Could you check a few things on this model? Use its own coordinates, in mm. Face numbers are marked on the shaded views. A direction names the side the tool comes from. Coordinates: 2 decimals unless noted, no trailing zeros. Loops run counter-clockwise (first coordinate to the right, second up) from the corner with the lowest first, then second, coordinate; pieces in that order, holes last. Notation, with made-up numbers: M 78,33 L 128,33 A16 cw 128,45 Z; hole C -5.5,-36.5 d11. An arc over 180 degrees is marked long. Use one line per item in the form item = value. Start each with the question number.
```python
from build123d import *

# Parameters (mm, degrees)
F0_R     = 10.5
F1_DEPTH = 6.35


with BuildPart() as f1:
    # F0 (on Top) → F1 (new body)
    with BuildSketch(Plane.XY):
        with BuildLine():
            ThreePointArc((6.44846, 29.992483), (-15.414201, 40.590403), (-10.190932, 16.862585))
            ThreePointArc((-10.190932, 16.862585), (-3.961799, 16.850813), (1.609508, 19.63699))
            ThreePointArc((1.609508, 19.63699), (5.17904, 24.277334), (6.44846, 29.992483))
        make_face()
        with Locations((-7.05154, 29.992483)):
            Circle(F0_R, mode=Mode.SUBTRACT)
        with BuildLine():
            Line((-14.895684, -5.7813), (-6.689736, -14.510419))
            ThreePointArc((-6.689736, -14.510419), (3.65694, -15.554151), (12.454594, -10.00939))
            Line((12.454594, -10.00939), (16.201378, -11.21237))
            ThreePointArc((16.201378, -11.21237), (16.574131, -4.994388), (19.698893, 0.394313))
            Line((19.698893, 0.394313), (15.911259, 1.461728))
            ThreePointArc((15.911259, 1.461728), (11.64182, 10.944078), (2.441089, 15.79069))
            Line((2.441089, 15.79069), (1.609508, 19.63699))
            ThreePointArc((1.609508, 19.63699), (-3.961799, 16.850813), (-10.190932, 16.862585))
            Line((-10.190932, 16.862585), (-9.221523, 13.048691))
            ThreePointArc((-9.221523, 13.048691), (-15.29876, 4.610072), (-14.895684, -5.7813))
        make_face()
        Circle(F0_R, mode=Mode.SUBTRACT)
        with BuildLine():
            Line((-9.507961, -17.256899), (-6.689736, -14.510419))
            Line((-6.689736, -14.510419), (-14.895684, -5.7813))
            Line((-14.895684, -5.7813), (-17.810886, -8.42462))
            ThreePointArc((-17.810886, -8.42462), (-12.612333, -11.856425), (-9.507961, -17.256899))
        make_face()
        with BuildLine():
            ThreePointArc((19.698893, 0.394313), (16.574131, -4.994388), (16.201378, -11.21237))
            ThreePointArc((16.201378, -11.21237), (30.665848, -22.338996), (43.000022, -8.889429))
            ThreePointArc((43.000022, -8.889429), (34.496759, 3.651808), (19.698893, 0.394313))
        make_face()
        with Locations((29.500022, -8.889429)):
            Circle(F0_R, mode=Mode.SUBTRACT)
        with BuildLine():
            ThreePointArc((-8.948482, -21.103054), (-9.089084, -19.159737), (-9.507961, -17.256899))
            ThreePointArc((-9.507961, -17.256899), (-12.612333, -11.856425), (-17.810886, -8.42462))
            ThreePointArc((-17.810886, -8.42462), (-33.513236, -28.837472), (-8.948482, -21.103054))
        make_face()
        with Locations((-22.448482, -21.103054)):
            Circle(F0_R, mode=Mode.SUBTRACT)
    extrude(amount=F1_DEPTH)


solid = f1.part
```
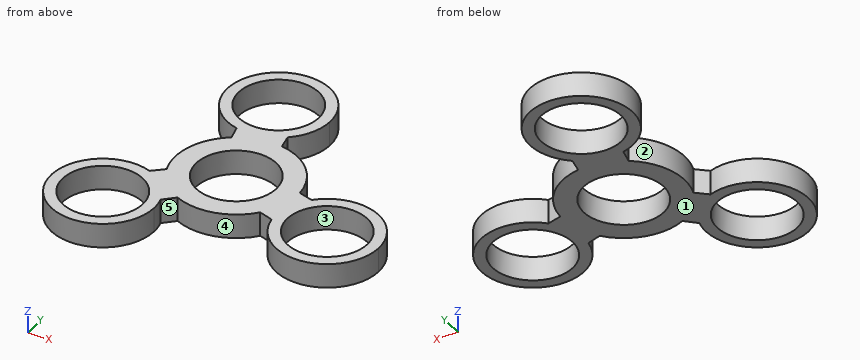
Item 1: I want a section at C-C (z = 4.5). Write out the boundary of the cut face in (x, y), plus the area to 3 significant figures.
Item 2: Thinking about a two-plate mould opening in X: for the marked faces 1, 2 and 3, which applies, pulls with the +X half, pulls with the -X half, needs draft (parallel to the pull), parting line crosses it, or undercut?
Item 3: I'm going to push flat-ended pins straight in: P1, Ø17, axis at x = -22.45, y = -21.1, coming from the +Z side; P2, Ø3, axis at y = -10, z = 4, coming from the -X side; P3, Ø1, axis at y = 11, z = 0.5, coming from the -X side. Where does each tip first touch, or does it pass through?
Item 4: I want a section at D-D (x = 0). Write out the boundary of the cut face in (y, z).
Item 5: I want a section at B-B (y = 28.5). Write out the boundary of the cut face in (x, z), plus the area to 3 significant figures.
Item 6: For the marked faces 4 and 5, which set-ups out of +Z, -Z, +X, -X, +Y, -Y let a thin tool reach every point of the face, with its end or its side?
Item 7: I want a section at A-A (x = 29.5). Write out the boundary of the cut face in (y, z), plus the area to 3 significant figures.
Item 8: Please list where these lines run through material, in increasing order: line 1 along Y through (x, z) = (-6, 6); line 2 along Y through (x, z) = (-1, 3.75); line 3 along X through (y, z) = (-20.5, 4.5) (3 decimals).
Worked answers:
q1.outline = M -17.81,-8.42 A13.5 ccw long -9.51,-17.26 L -6.69,-14.51 A15.98 ccw 12.45,-10.01 L 16.2,-11.21 A13.5 ccw long 19.7,0.39 L 15.91,1.46 A15.98 ccw 2.44,15.79 L 1.61,19.64 A13.5 ccw 6.45,29.99 A13.5 ccw long -10.19,16.86 L -9.22,13.05 A15.98 ccw -14.9,-5.78 Z; hole C -22.45,-21.1 d21; hole C -7.05,29.99 d21; hole C 0,0 d21; hole C 29.5,-8.89 d21
q1.area = 1,210 mm²
q2.face_1 = needs draft
q2.face_2 = pulls with the -X half
q2.face_3 = undercut
q3.P1 = through
q3.P2 = -31.94
q3.P3 = -12.04
q4.outline = M -15.98,0 L -10.5,0 L -10.5,6.35 L -15.98,6.35 Z; M 10.5,0 L 22.21,0 L 22.21,6.35 L 10.5,6.35 Z; M 37.77,0 L 41.5,0 L 41.5,6.35 L 37.77,6.35 Z
q5.outline = M -20.47,0 L -17.44,0 L -17.44,6.35 L -20.47,6.35 Z; M 3.34,0 L 6.37,0 L 6.37,6.35 L 3.34,6.35 Z
q5.area = 38.4 mm²
q6.face_4 = +Z, -Z, -Y
q6.face_5 = +Z, -Z
q7.outline = M -22.39,0 L -19.39,0 L -19.39,6.35 L -22.39,6.35 Z; M 1.61,0 L 4.61,0 L 4.61,6.35 L 1.61,6.35 Z
q7.area = 38.1 mm²
q8.line_1 = -14.81 to -8.62, 8.62 to 19.55, 40.44 to 43.45
q8.line_2 = -15.95 to -10.45, 10.45 to 21.41, 38.57 to 42.06
q8.line_3 = -35.935 to -32.931, -11.966 to -8.962, 22.612 to 36.388
